Model file for the job. Use its own axes, mm. Face numbers are marked on the shaded views. A direction names the side the tool comes from. Round coordinates to 2 decimals unless told otherwise and drop trailing zeros. Order: outer loops, then holes, each group sorted by start corner. A loop starts at its lowest first (then second) coordinate and runs counter-clockwise, first axis right, second up. Notation, with made-up numbers: (42, 22) - (55, 22) arc R18 cw to (55, 57) - close; hole circle Ø8 at (-4, 75.5). An arc over 180 degrees is marked (long way). Answer as CSV lines item,"result". Start each with the question number.
1. Pin check, flat tips, straight feed: pin 1 Ø5 at (x, z) = (-0.5, -7.5) entering from +Y; pin 2 Ø1.1 at (y, z) = (4, 21.5) entering from +X; pin 3 Ø1 at (x, y) = (7, 29) entering from +Z. Stop position of each tip, or through.
2. Pull direction Y, two halves, no side cores. Call the marked faces 1, 2 and 3: released by +Y, released by -Y, zero draft, split by the parting line, or undercut.
3. Wall check: line 1 along Z through (x, y) = (15.6, 42.5); line 2 along Z through (x, y) = (12, 16.5). Give the ranges that are in metal, low to high. Write a range as [from, to].
4. Band-saw the part on B-B on z = 18. List the corners of the cut face in (x, y), then the cut area to 3 significant figures.
5. Band-saw the part on C-C on y = 16. List the corners of the cut face in (x, z).
6. Band-saw the part on D-D on x = 0. List the corners of the cut face in (y, z).
7. Band-saw the part on A-A on y = 47. List the corners of the cut face in (x, z), then the cut area to 3 significant figures.
8. 3-axis set-ups, long thin cutter, end or side, ignore diameter. For the marked faces 4, 5 and 6: which of +Z, -Z, +X, -X, +Y, -Y reach the whole face in a straight line?
```python
from build123d import *

# Parameters (mm, degrees)
SKETCH1_W               = 42.3
SKETCH1_H               = 42.3
BOSS_EXTRUDE1_DEPTH     = 48
SKETCH2_R               = 11.5
BOSS_EXTRUDE2_DEPTH     = 2
SKETCH3_R               = 2.5
BOSS_EXTRUDE3_DEPTH     = 23
SKETCH4_R               = 1.5
CUT_EXTRUDE1_DEPTH      = 8
MIRROR3_COPY_1_SKETCH_R = 1.5
MIRROR3_COPY_1_DEPTH    = 8
CUT_EXTRUDE2_DEPTH      = 9.5
MIRROR5_COPY_1_DEPTH    = 9.5
SKETCH7_R               = 2.5
CUT_EXTRUDE5_DEPTH      = 5
CUT_EXTRUDE6_DEPTH      = 11
MIRROR7_COPY_1_DEPTH    = 11
CUT_EXTRUDE7_DEPTH      = 27.5
CUT_EXTRUDE8_DEPTH      = 27.5
CUT_EXTRUDE9_DEPTH      = 27.5
CUT_EXTRUDE10_DEPTH     = 27.5
BOSS_EXTRUDE4_DEPTH     = 1


with BuildPart() as part:
    # Sketch1 → Boss-Extrude1 (new body)
    with BuildSketch(Plane(origin=(0, 0, 0), x_dir=(1, 0, 0), z_dir=(0, 1, 0))):
        Rectangle(SKETCH1_W, SKETCH1_H)
    extrude(amount=BOSS_EXTRUDE1_DEPTH)

    # Sketch2 → Boss-Extrude2 (add)
    with BuildSketch(Plane(origin=(0, 48, 0), x_dir=(1, 0, 0), z_dir=(0, 1, 0))):
        Circle(SKETCH2_R)
    extrude(amount=BOSS_EXTRUDE2_DEPTH)

    # Sketch3 → Boss-Extrude3 (add)
    with BuildSketch(Plane(origin=(0, 50, 0), x_dir=(1, 0, 0), z_dir=(0, 1, 0))):
        Circle(SKETCH3_R)
    extrude(amount=BOSS_EXTRUDE3_DEPTH)

    # Sketch4 → Cut-Extrude1 (cut)
    with BuildSketch(Plane(origin=(0, 48, 0), x_dir=(1, 0, 0), z_dir=(0, 1, 0))):
        with Locations((-15.6, 15.6)):
            Circle(SKETCH4_R)
    cut_extrude1 = extrude(amount=-CUT_EXTRUDE1_DEPTH, mode=Mode.SUBTRACT)

    # Mirror1: Cut-Extrude1 across plane
    add(cut_extrude1.mirror(Plane(origin=(0, 0, 0), x_dir=(0, 0, 1), z_dir=(1, 0, 0))), mode=Mode.SUBTRACT)

    # Mirror3: Cut-Extrude1 across plane
    add(cut_extrude1.mirror(Plane.XY), mode=Mode.SUBTRACT)

    # Mirror3 copy 1 sketch → Mirror3 copy 1 (cut)
    with BuildSketch(Plane(origin=(0, 48, 0), x_dir=(-1, 0, 0), z_dir=(0, 1, 0))):
        with Locations((-15.6, 15.6)):
            Circle(MIRROR3_COPY_1_SKETCH_R)
    extrude(amount=-MIRROR3_COPY_1_DEPTH, mode=Mode.SUBTRACT)

    # Sketch6 → Cut-Extrude2 (cut)
    with BuildSketch(Plane(origin=(0, 48, 0), x_dir=(1, 0, 0), z_dir=(0, 1, 0))):
        Polygon((-21.15, 21.15), (-21.15, 16.08), (-16.08, 21.15), align=None)
    cut_extrude2 = extrude(amount=-CUT_EXTRUDE2_DEPTH, mode=Mode.SUBTRACT)

    # Mirror4: Cut-Extrude2 across plane
    add(cut_extrude2.mirror(Plane(origin=(0, 0, 0), x_dir=(0, 0, 1), z_dir=(1, 0, 0))), mode=Mode.SUBTRACT)

    # Mirror5: Cut-Extrude2 across plane
    add(cut_extrude2.mirror(Plane.XY), mode=Mode.SUBTRACT)

    # Mirror5 copy 1 sketch → Mirror5 copy 1 (cut)
    with BuildSketch(Plane(origin=(0, 48, 0), x_dir=(-1, 0, 0), z_dir=(0, 1, 0))):
        Polygon((-21.15, 21.15), (-21.15, 16.08), (-16.08, 21.15), align=None)
    extrude(amount=-MIRROR5_COPY_1_DEPTH, mode=Mode.SUBTRACT)

    # Sketch7 → Cut-Extrude5 (cut)
    with BuildSketch(Plane.XZ):
        Circle(SKETCH7_R)
    extrude(amount=-CUT_EXTRUDE5_DEPTH, mode=Mode.SUBTRACT)

    # Sketch8 → Cut-Extrude6 (cut)
    with BuildSketch(Plane.XZ):
        Polygon((-21.15, 21.15), (-21.15, 16.08), (-16.08, 21.15), align=None)
    cut_extrude6 = extrude(amount=-CUT_EXTRUDE6_DEPTH, mode=Mode.SUBTRACT)

    # Mirror6: Cut-Extrude6 across plane
    add(cut_extrude6.mirror(Plane(origin=(0, 0, 0), x_dir=(0, 0, 1), z_dir=(1, 0, 0))), mode=Mode.SUBTRACT)

    # Mirror7: Cut-Extrude6 across plane
    add(cut_extrude6.mirror(Plane.XY), mode=Mode.SUBTRACT)

    # Mirror7 copy 1 sketch → Mirror7 copy 1 (cut)
    with BuildSketch(Plane(origin=(0, 0, 0), x_dir=(-1, 0, 0), z_dir=(0, -1, 0))):
        Polygon((-21.15, 21.15), (-21.15, 16.08), (-16.08, 21.15), align=None)
    extrude(amount=-MIRROR7_COPY_1_DEPTH, mode=Mode.SUBTRACT)

    # Sketch10 → Cut-Extrude7 (cut)
    with BuildSketch(Plane(origin=(0, 38.5, 0), x_dir=(1, 0, 0), z_dir=(0, 1, 0))):
        Polygon((-21.15, 21.15), (-12.15, 21.15), (-21.15, 12.15), align=None)
    extrude(amount=-CUT_EXTRUDE7_DEPTH, mode=Mode.SUBTRACT)

    # Sketch11 → Cut-Extrude8 (cut)
    with BuildSketch(Plane(origin=(0, 38.5, 0), x_dir=(1, 0, 0), z_dir=(0, 1, 0))):
        Polygon((21.15, 21.15), (12.15, 21.15), (21.15, 12.15), align=None)
    extrude(amount=-CUT_EXTRUDE8_DEPTH, mode=Mode.SUBTRACT)

    # Sketch12 → Cut-Extrude9 (cut)
    with BuildSketch(Plane(origin=(0, 38.5, 0), x_dir=(1, 0, 0), z_dir=(0, 1, 0))):
        Polygon((-21.15, -21.15), (-12.15, -21.15), (-21.15, -12.15), align=None)
    extrude(amount=-CUT_EXTRUDE9_DEPTH, mode=Mode.SUBTRACT)

    # Sketch13 → Cut-Extrude10 (cut)
    with BuildSketch(Plane(origin=(0, 38.5, 0), x_dir=(1, 0, 0), z_dir=(0, 1, 0))):
        Polygon((21.15, -21.15), (21.15, -12.15), (12.15, -21.15), align=None)
    extrude(amount=-CUT_EXTRUDE10_DEPTH, mode=Mode.SUBTRACT)

    # Sketch14 → Boss-Extrude4 (add)
    with BuildSketch(Plane.XY.offset(21.15)):
        Polygon((0, 0), (-3, 0), (-3, 9), (3, 9), (3, 0), align=None)
    extrude(amount=BOSS_EXTRUDE4_DEPTH)


solid = part.part
```
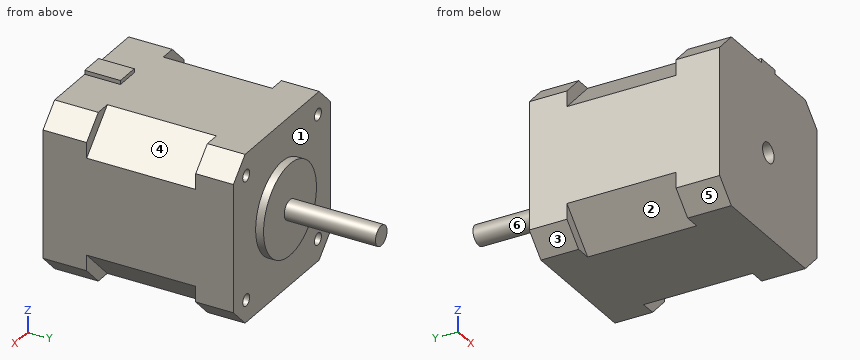
Reply:
1,pin 1,"stops at y = 50"
1,pin 2,"stops at x = 16.28"
1,pin 3,"stops at z = 21.15"
2,face 1,"released by +Y"
2,face 2,"undercut"
2,face 3,"zero draft"
3,line 1,"z = [-21.15, -17.1], [-14.1, 14.1], [17.1, 21.15]"
3,line 2,"z = [-21.15, 21.15]"
4,outline,"(-19.23, 0) - (19.23, 0) - (19.23, 11) - (15.3, 11) - (15.3, 38.5) - (19.23, 38.5) - (19.23, 48) - (-19.23, 48) - (-19.23, 38.5) - (-15.3, 38.5) - (-15.3, 11) - (-19.23, 11) - close"
4,area,"1,630 mm2"
5,outline,"(-21.15, -12.15) - (-12.15, -21.15) - (12.15, -21.15) - (21.15, -12.15) - (21.15, 12.15) - (12.15, 21.15) - (-12.15, 21.15) - (-21.15, 12.15) - close"
6,outline,"(0, -21.15) - (48, -21.15) - (48, -11.5) - (50, -11.5) - (50, -2.5) - (73, -2.5) - (73, 2.5) - (50, 2.5) - (50, 11.5) - (48, 11.5) - (48, 21.15) - (9, 21.15) - (9, 22.15) - (0, 22.15) - (0, 2.5) - (5, 2.5) - (5, -2.5) - (0, -2.5) - close"
7,outline,"(-21.15, -16.08) - (-16.08, -21.15) - (16.08, -21.15) - (21.15, -16.08) - (21.15, 16.08) - (16.08, 21.15) - (-16.08, 21.15) - (-21.15, 16.08) - close; hole circle Ø3 at (-15.6, -15.6); hole circle Ø3 at (-15.6, 15.6); hole circle Ø3 at (15.6, -15.6); hole circle Ø3 at (15.6, 15.6)"
7,area,"1,710 mm2"
8,face 4,"+Z, +X"
8,face 5,"-Z, -X, +Y, -Y"
8,face 6,"+Y"
